from build123d import *

# Parameters (mm, degrees)
SKETCH1_W           = 8
SKETCH1_H           = 6
BOSS_EXTRUDE1_DEPTH = 10
SKETCH3_W           = 26
SKETCH3_H           = 6
SKETCH3_R           = 1
BOSS_EXTRUDE2_DEPTH = 1.8
SKETCH4_W           = 5.9
SKETCH4_H           = 3.2
CUT_EXTRUDE1_DEPTH  = 7
CUT_EXTRUDE2_START  = -4
SKETCH6_R           = 1
CUT_EXTRUDE2_DEPTH  = 4


with BuildPart() as part:
    # Sketch1 → Boss-Extrude1 (new body)
    with BuildSketch(Plane(origin=(0, 0, 0), x_dir=(1, 0, 0), z_dir=(0, 1, 0))):
        with Locations((-4, 3)):
            Rectangle(SKETCH1_W, SKETCH1_H)
    extrude(amount=BOSS_EXTRUDE1_DEPTH)

    # Sketch3 → Boss-Extrude2 (add)
    with BuildSketch(Plane(origin=(0, 10, 0), x_dir=(1, 0, 0), z_dir=(0, 1, 0))):
        with Locations((-11, 3)):
            Rectangle(SKETCH3_W, SKETCH3_H)
        with Locations(Location((-20.5, 3, 0), (0, 0, 270))):
            Circle(SKETCH3_R, mode=Mode.SUBTRACT)
        with Locations(Location((-1.5, 3, 0), (0, 0, 90))):
            Circle(SKETCH3_R, mode=Mode.SUBTRACT)
    extrude(amount=BOSS_EXTRUDE2_DEPTH)

    # Sketch4 → Cut-Extrude1 (cut)
    with BuildSketch(Plane.XZ):
        with Locations((-4, -3)):
            Rectangle(SKETCH4_W, SKETCH4_H)
    extrude(amount=-CUT_EXTRUDE1_DEPTH, mode=Mode.SUBTRACT)

    # Sketch6 → Cut-Extrude2 (cut)
    with BuildSketch(Plane(origin=(0, 11.8, 0), x_dir=(1, 0, 0), z_dir=(0, 1, 0)).offset(CUT_EXTRUDE2_START)):
        with Locations(Location((-1.5, 3, 0), (0, 0, 90))):
            Circle(SKETCH6_R)
    extrude(amount=CUT_EXTRUDE2_DEPTH, mode=Mode.SUBTRACT)


solid = part.part
Design review of the part built by this model. Coordinates are the model's own, in mm. A direction names the side the tool comes from. Give positions to 0.01 mm unless a question says otherwise; leave off trailing zeros. Loops run counter-clockwise (first coordinate to the right, second up) from the corner with the lowest first, then second, coordinate; pieces in that order, holes last. Notation, with made-up numbers: (-18, 2) - (5, 2) arc R21 cw to (5, 17) - close; hole circle Ø7 at (30.5, 5.25). An arc over 180 degrees is marked (long way). Write item = value, one per line.
1) Take a section at B-B on x = -20.5. State the section outline as (y, z) points, and give its area (3 significant figures).
Result sheet:
outline = (10, -6) - (11.8, -6) - (11.8, -4) - (10, -4) - close; (10, -2) - (11.8, -2) - (11.8, 0) - (10, 0) - close
area = 7.20 mm2
2) Tool access review of faces 1 (the face through (-16, 10, -3)), 2 (the face through (-0.9, 9.8, -2.2)), 3 (the face through (-4, 7, -3)): name each direction out of +Z, -Z, +X, -X, +Y, -Y from which nothing blocks a thin tool from reaching the whole face with its end or side.
Result sheet:
face_1 = +Z, -Z, -X, -Y
face_2 = +Y
face_3 = -Y
3) Take a section at D-D on x = -2.75. State the section outline as (y, z) points.
Result sheet:
outline = (0, -6) - (11.8, -6) - (11.8, 0) - (0, 0) - (0, -1.4) - (7, -1.4) - (7, -4.6) - (0, -4.6) - close
4) Draft analysis for pull direction Z (two halves, no side actions). For faces 4 (the face through (-21.476, 10.887, -3.217)), 5 (the face through (1, 10, -3)), 6 (the face through (-6, 8, 0)), state which applies: +Z half, -Z half, draft (parallel to the pull), parting line (faces both ways), or undercut.
Result sheet:
face_4 = undercut
face_5 = draft
face_6 = +Z half
5) Take a section at C-C on z = -1.1. State the section outline as (x, y) points.
Result sheet:
outline = (-24, 10) - (-8, 10) - (-8, 0) - (0, 0) - (0, 10) - (2, 10) - (2, 11.8) - (-24, 11.8) - close
6) Take a section at A-A on z = -3. State the section outline as (x, y) points.
Result sheet:
outline = (-24, 10) - (-21.5, 10) - (-21.5, 11.8) - (-24, 11.8) - close; (-19.5, 10) - (-8, 10) - (-8, 0) - (-6.95, 0) - (-6.95, 7) - (-1.05, 7) - (-1.05, 0) - (0, 0) - (0, 10) - (2, 10) - (2, 11.8) - (-0.5, 11.8) - (-0.5, 7.8) - (-2.5, 7.8) - (-2.5, 11.8) - (-19.5, 11.8) - close
7) To check wall thickness, follow line 1 (X direction, y = 10.9, z = -3); line 2 (X direction, y = 6.25, z = -3.6); line 3 (Z direction, x = -2.25, y = 2.25). State the ranges of each line that lie inside material, in increasing order.
Result sheet:
line_1 = -24 to -21.5, -19.5 to -2.5, -0.5 to 2
line_2 = -8 to -6.95, -1.05 to 0
line_3 = -6 to -4.6, -1.4 to 0
8) Clearance check with flat-ended pins moving along their axes: pin 1 Ø1.6 at (y, z) = (2.5, -3) entering from +X; pin 2 Ø2.5 at (x, z) = (-4.5, -3) entering from -Y; pin 3 Ø3 at (y, z) = (4, -2) entering from -X; pin 4 Ø1.6 at (x, z) = (-20.5, -3) entering from +Y. State where each tip first meets the part, or that it passes through.
Result sheet:
pin_1 = 0
pin_2 = 7
pin_3 = -8
pin_4 = through
